Design review of the part built by this model. Coordinates are the model's own, in mm. A direction names the side the tool comes from. Give positions to 0.01 mm unless a question says otherwise; leave off trailing zeros. Loops run counter-clockwise (first coordinate to the right, second up) from the corner with the lowest first, then second, coordinate; pieces in that order, holes last.
from build123d import *

# Parameters (mm, degrees)
ESQUISSE1_W              = 44
ESQUISSE1_H              = 25
BOSS_EXTRU_1_DEPTH       = 1.9
ESQUISSE2_W              = 18
ESQUISSE2_H              = 21.4
ESQUISSE2_W_2            = 12.9
ESQUISSE2_H_2            = 20.7
ENL_V_MAT_EXTRU_1_DEPTH  = 1.1
ESQUISSE3_W              = 9
ESQUISSE3_H              = 12
ENL_V_MAT_EXTRU_2_DEPTH  = 10
ESQUISSE4_W              = 3.5
ESQUISSE4_H              = 6.801352385
ENL_V_MAT_EXTRU_3_DEPTH  = 1.4
ENL_V_MAT_EXTRU_4_DEPTH  = 2.4
ESQUISSE6_W              = 9
ESQUISSE6_H              = 0.8
BOSS_EXTRU_2_DEPTH       = 1
ESQUISSE7_W              = 2
ESQUISSE7_H              = 1.1
BOSS_EXTRU_3_DEPTH       = 1
BOSS_EXTRU_4_DEPTH       = 1
ESQUISSE12_W             = 26.5
ESQUISSE12_H             = 1.9
BOSS_EXTRU_6_DEPTH       = 1
ESQUISSE13_W             = 44
ESQUISSE13_H             = 1
BOSS_EXTRU_7_DEPTH       = 4.9
ESQUISSE14_W             = 44
ESQUISSE14_H             = 27
BOSS_EXTRU_8_DEPTH       = 0.8
ESQUISSE15_W             = 9
ESQUISSE15_H             = 1
ENL_V_MAT_EXTRU_5_DEPTH  = 0.2
ESQUISSE16_W             = 0.8
ESQUISSE16_H             = 1.1
ENL_V_MAT_EXTRU_7_DEPTH  = 2
ESQUISSE18_W             = 1.9
ESQUISSE18_H             = 3.15
ENL_V_MAT_EXTRU_8_DEPTH  = 2
ESQUISSE19_W             = 1
ESQUISSE19_H             = 25
BOSS_EXTRU_10_DEPTH      = 4.9
ENL_V_MAT_EXTRU_9_DEPTH  = 1
ESQUISSE21_W             = 1.9
ESQUISSE21_H             = 2.150656269
BOSS_EXTRU_11_DEPTH      = 17.5
BOSS_EXTRU_12_DEPTH      = 1.1
BOSS_EXTRU_13_DEPTH      = 1.1
ESQUISSE26_W             = 12.9
ESQUISSE26_H             = 17.5
ENL_V_MAT_EXTRU_10_DEPTH = 1.1
ESQUISSE28_W             = 4.9
ESQUISSE28_H             = 25
ENL_V_MAT_EXTRU_12_DEPTH = 10
ESQUISSE30_W             = 4.9
ESQUISSE30_H             = 25
BOSS_EXTRU_14_DEPTH      = 1
ESQUISSE31_W             = 4.9
ESQUISSE31_H             = 4.778042902
ESQUISSE31_H_2           = 4.777647835
ENL_V_MAT_EXTRU_13_DEPTH = 11
ESQUISSE32_W             = 2
ESQUISSE32_H             = 1.1
ENL_V_MAT_EXTRU_14_DEPTH = 5
ESQUISSE33_W             = 4.880014168
ESQUISSE33_H             = 9.610289291
ENL_V_MAT_EXTRU_15_DEPTH = 5
ESQUISSE34_W             = 1.1
ESQUISSE34_H             = 10.612062874
ENL_V_MAT_EXTRU_16_DEPTH = 5
ESQUISSE35_W             = 1.1
ESQUISSE35_H             = 16.502088347
BOSS_EXTRU_15_DEPTH      = 0.1
ESQUISSE36_W             = 1.95
ESQUISSE36_H             = 2.065080621
ESQUISSE36_W_2           = 1.843442291
BOSS_EXTRU_16_DEPTH      = 1
ESQUISSE40_W             = 3.7
ESQUISSE40_H             = 6.2
ENL_V_MAT_EXTRU_18_DEPTH = 1
ESQUISSE39_W             = 7.2
ESQUISSE39_H             = 3
ENL_V_MAT_EXTRU_20_DEPTH = 1
ESQUISSE41_W             = 1.072034993
ESQUISSE41_H             = 2.997764605
ESQUISSE41_W_2           = 1.033542433
BOSS_EXTRU_17_DEPTH      = 0.2
ESQUISSE42_W             = 1.1
ESQUISSE42_H             = 9.602531403
ENL_V_MAT_EXTRU_21_DEPTH = 0.2


with BuildPart() as part:
    # Esquisse1 → Boss.-Extru.1 (new body)
    with BuildSketch(Plane.XY):
        Rectangle(ESQUISSE1_W, ESQUISSE1_H)
    extrude(amount=BOSS_EXTRU_1_DEPTH)

    # Esquisse2 → Enlèv. mat.-Extru.1 (cut)
    with BuildSketch(Plane.XY.offset(1.9)):
        with Locations((-11.5, 1.801352385)):
            Rectangle(ESQUISSE2_W, ESQUISSE2_H)
        with Locations((12.55, -0.999343731)):
            Rectangle(ESQUISSE2_W_2, ESQUISSE2_H_2)
    extrude(amount=-ENL_V_MAT_EXTRU_1_DEPTH, mode=Mode.SUBTRACT)

    # Esquisse3 → Enlèv. mat.-Extru.2 (cut)
    with BuildSketch(Plane.XY.offset(0.8)):
        with Locations((-11.5, 12.5)):
            Rectangle(ESQUISSE3_W, ESQUISSE3_H)
    extrude(amount=-ENL_V_MAT_EXTRU_2_DEPTH, mode=Mode.SUBTRACT)

    # Esquisse4 → Enlèv. mat.-Extru.3 (cut)
    with BuildSketch(Plane.XY.offset(1.9)):
        with Locations((-6.25, -9.099323807)):
            Rectangle(ESQUISSE4_W, ESQUISSE4_H)
    extrude(amount=-ENL_V_MAT_EXTRU_3_DEPTH, mode=Mode.SUBTRACT)

    # Esquisse5 → Enlèv. mat.-Extru.4 (cut)
    with BuildSketch(Plane.XY.offset(1.9)):
        Polygon((-8, -5.698647615), (-14.25, -8.898647615), (-22, -8.898647615), (-22, -12.5), (-4.5, -12.5), (-4.5, -5.698647615), align=None)
    extrude(amount=-ENL_V_MAT_EXTRU_4_DEPTH, mode=Mode.SUBTRACT)

    # Esquisse6 → Boss.-Extru.2 (add)
    with BuildSketch(Plane(origin=(0, 6.5, 0), x_dir=(1, 0, 0), z_dir=(0, 1, 0))):
        with Locations((-11.5, -0.4)):
            Rectangle(ESQUISSE6_W, ESQUISSE6_H)
    extrude(amount=BOSS_EXTRU_2_DEPTH)

    # Esquisse7 → Boss.-Extru.3 (add)
    with BuildSketch(Plane(origin=(0, -8.898647615, 0), x_dir=(1, 0, 0), z_dir=(0, 1, 0))):
        with Locations((-3.5, -1.35)):
            Rectangle(ESQUISSE7_W, ESQUISSE7_H)
    extrude(amount=BOSS_EXTRU_3_DEPTH)

    # Esquisse9 → Boss.-Extru.4 (add)
    with BuildSketch(Plane(origin=(0, 12.5, 0), x_dir=(1, 0, 0), z_dir=(0, 1, 0))):
        Polygon((22, 0), (-2.5, 0), (-7, 0), (-7, -0.8), (-2.5, -0.8), (-2.5, -1.9), (22, -1.9), align=None)
        Polygon((-22, 0), (-20.5, 0), (-16, 0), (-16, -0.8), (-20.5, -0.8), (-20.5, -1.9), (-22, -1.9), align=None)
    extrude(amount=BOSS_EXTRU_4_DEPTH)

    # Esquisse12 → Boss.-Extru.6 (add)
    with BuildSketch(Plane.XZ.offset(12.5)):
        with Locations((8.75, 0.95)):
            Rectangle(ESQUISSE12_W, ESQUISSE12_H)
    extrude(amount=BOSS_EXTRU_6_DEPTH)

    # Esquisse13 → Boss.-Extru.7 (add)
    with BuildSketch(Plane(origin=(0, 0, 0), x_dir=(-1, 0, 0), z_dir=(0, 0, -1))):
        with Locations((0, 13)):
            Rectangle(ESQUISSE13_W, ESQUISSE13_H)
        with Locations((0, -13)):
            Rectangle(ESQUISSE13_W, ESQUISSE13_H)
    extrude(amount=BOSS_EXTRU_7_DEPTH)

    # Esquisse14 → Boss.-Extru.8 (add)
    with BuildSketch(Plane(origin=(0, 0, -4.9), x_dir=(-1, 0, 0), z_dir=(0, 0, -1))):
        Rectangle(ESQUISSE14_W, ESQUISSE14_H)
    extrude(amount=BOSS_EXTRU_8_DEPTH)

    # Esquisse15 → Enlèv. mat.-Extru.5 (cut)
    with BuildSketch(Plane.XY):
        with Locations((-11.5, 13)):
            Rectangle(ESQUISSE15_W, ESQUISSE15_H)
    extrude(amount=-ENL_V_MAT_EXTRU_5_DEPTH, mode=Mode.SUBTRACT)

    # Esquisse16 → Enlèv. mat.-Extru.7 (cut)
    with BuildSketch(Plane.ZY.offset(22)):
        with Locations((-5.3, 11.95)):
            Rectangle(ESQUISSE16_W, ESQUISSE16_H)
    extrude(amount=-ENL_V_MAT_EXTRU_7_DEPTH, mode=Mode.SUBTRACT)

    # Esquisse18 → Enlèv. mat.-Extru.8 (cut)
    with BuildSketch(Plane(origin=(22, 0, 0), x_dir=(0, 0, -1), z_dir=(1, 0, 0))):
        with Locations((-0.95, 10.925)):
            Rectangle(ESQUISSE18_W, ESQUISSE18_H)
    extrude(amount=-ENL_V_MAT_EXTRU_8_DEPTH, mode=Mode.SUBTRACT)

    # Esquisse19 → Boss.-Extru.10 (add)
    with BuildSketch(Plane.XY.offset(-4.9)):
        with Locations((-19.5, 0)):
            Rectangle(ESQUISSE19_W, ESQUISSE19_H)
    extrude(amount=BOSS_EXTRU_10_DEPTH)

    # Esquisse20 → Enlèv. mat.-Extru.9 (cut)
    with BuildSketch(Plane.XY.offset(0.8)):
        Polygon((-4.5, -5.776745759), (-4.5, -3.002088347), (-8.02831202, -3.002088347), (-11.125, -7.298647615), align=None)
    extrude(amount=-ENL_V_MAT_EXTRU_9_DEPTH, mode=Mode.SUBTRACT)

    # Esquisse21 → Boss.-Extru.11 (add)
    with BuildSketch(Plane.ZY.offset(4.5)):
        with Locations((0.95, -12.424671866)):
            Rectangle(ESQUISSE21_W, ESQUISSE21_H)
    extrude(amount=BOSS_EXTRU_11_DEPTH)

    # Esquisse23 → Boss.-Extru.12 (add)
    with BuildSketch(Plane.XY.offset(0.8)):
        Polygon((-4.5, -7.898647615), (-11.348803677, -11.349343731), (-4.5, -11.349343731), align=None)
    extrude(amount=BOSS_EXTRU_12_DEPTH)

    # Esquisse25 → Boss.-Extru.13 (add)
    with BuildSketch(Plane.XY.offset(0.8)):
        Polygon((-16, 13.5), (-20.5, 13.5), (-20.5, -8.898647615), (-14.25, -8.898647615), (-11.125, -7.298647615), (-8.02831202, -3.002088347), (-4.5, -3.002088347), (-4.5, -7.898647615), (-2.5, -7.898647615), (-2.5, 13.5), (-7, 13.5), (-7, 7.5), (-16, 7.5), align=None)
    extrude(amount=BOSS_EXTRU_13_DEPTH)

    # Esquisse26 → Enlèv. mat.-Extru.10 (cut)
    with BuildSketch(Plane.XY.offset(1.9)):
        with Locations((-11.5, 4.75)):
            Rectangle(ESQUISSE26_W, ESQUISSE26_H)
    extrude(amount=-ENL_V_MAT_EXTRU_10_DEPTH, mode=Mode.SUBTRACT)

    # Esquisse28 → Enlèv. mat.-Extru.12 (cut)
    with BuildSketch(Plane.ZY.offset(20)):
        with Locations((-2.45, 0)):
            Rectangle(ESQUISSE28_W, ESQUISSE28_H)
    extrude(amount=-ENL_V_MAT_EXTRU_12_DEPTH, mode=Mode.SUBTRACT)

    # Esquisse30 → Boss.-Extru.14 (add)
    with BuildSketch(Plane.ZY.offset(22)):
        with Locations((-2.45, 0)):
            Rectangle(ESQUISSE30_W, ESQUISSE30_H)
    extrude(amount=-BOSS_EXTRU_14_DEPTH)

    # Esquisse31 → Enlèv. mat.-Extru.13 (cut)
    with BuildSketch(Plane(origin=(-21, 0, 0), x_dir=(0, 0, -1), z_dir=(1, 0, 0))):
        with Locations((2.45, 10.110978549)):
            Rectangle(ESQUISSE31_W, ESQUISSE31_H)
        with Locations((2.45, -10.111176083)):
            Rectangle(ESQUISSE31_W, ESQUISSE31_H_2)
    extrude(amount=-ENL_V_MAT_EXTRU_13_DEPTH, mode=Mode.SUBTRACT)

    # Esquisse32 → Enlèv. mat.-Extru.14 (cut)
    with BuildSketch(Plane(origin=(0, 0, -5.7), x_dir=(-1, 0, 0), z_dir=(0, 0, -1))):
        with Locations((21, 9.515350227)):
            Rectangle(ESQUISSE32_W, ESQUISSE32_H)
        with Locations((21, 6.785575873)):
            Rectangle(ESQUISSE32_W, ESQUISSE32_H)
    extrude(amount=-ENL_V_MAT_EXTRU_14_DEPTH, mode=Mode.SUBTRACT)

    # Esquisse33 → Enlèv. mat.-Extru.15 (cut)
    with BuildSketch(Plane.ZY.offset(22)):
        with Locations((-2.440007084, 7.694855354)):
            Rectangle(ESQUISSE33_W, ESQUISSE33_H)
    extrude(amount=-ENL_V_MAT_EXTRU_15_DEPTH, mode=Mode.SUBTRACT)

    # Esquisse34 → Enlèv. mat.-Extru.16 (cut)
    with BuildSketch(Plane.ZY.offset(22)):
        with Locations((-2.596187743, -2.416320728)):
            Rectangle(ESQUISSE34_W, ESQUISSE34_H)
    extrude(amount=-ENL_V_MAT_EXTRU_16_DEPTH, mode=Mode.SUBTRACT)

    # Esquisse35 → Boss.-Extru.15 (add)
    with BuildSketch(Plane.ZY.offset(5.05)):
        with Locations((1.35, 5.248955826)):
            Rectangle(ESQUISSE35_W, ESQUISSE35_H)
    extrude(amount=BOSS_EXTRU_15_DEPTH)

    # Esquisse36 → Boss.-Extru.16 (add)
    with BuildSketch(Plane.XY.offset(0.8)):
        with Locations((-16.975, 7.632540311)):
            Rectangle(ESQUISSE36_W, ESQUISSE36_H)
        with Locations((-6.078278855, 7.632540311)):
            Rectangle(ESQUISSE36_W_2, ESQUISSE36_H)
    extrude(amount=BOSS_EXTRU_16_DEPTH)

    # Esquisse40 → Enlèv. mat.-Extru.18 (cut)
    with BuildSketch(Plane.XY.offset(1.9)):
        with Locations((1.85, 0)):
            Rectangle(ESQUISSE40_W, ESQUISSE40_H)
    extrude(amount=-ENL_V_MAT_EXTRU_18_DEPTH, mode=Mode.SUBTRACT)

    # Esquisse39 → Enlèv. mat.-Extru.20 (cut)
    with BuildSketch(Plane.XY.offset(1.9)):
        with Locations((2.705958025, 12)):
            Rectangle(ESQUISSE39_W, ESQUISSE39_H)
    extrude(amount=-ENL_V_MAT_EXTRU_20_DEPTH, mode=Mode.SUBTRACT)

    # Esquisse41 → Boss.-Extru.17 (add)
    with BuildSketch(Plane.XY.offset(1.9)):
        with Locations((-1.430059472, 12.001117697)):
            Rectangle(ESQUISSE41_W, ESQUISSE41_H)
        with Locations((6.822729242, 12.001117697)):
            Rectangle(ESQUISSE41_W_2, ESQUISSE41_H)
    extrude(amount=BOSS_EXTRU_17_DEPTH)

    # Esquisse42 → Enlèv. mat.-Extru.21 (cut)
    with BuildSketch(Plane.ZY.offset(5.15)):
        with Locations((1.35, 1.799177355)):
            Rectangle(ESQUISSE42_W, ESQUISSE42_H)
    extrude(amount=-ENL_V_MAT_EXTRU_21_DEPTH, mode=Mode.SUBTRACT)


solid = part.part
Q1. Take a section at A-A (z = -4). Give the boundary of the cut face in (x, y), plus the area to 3 significant figures.
Results:
outline: (-22, -13.5) - (22, -13.5) - (22, -12.5) - (-22, -12.5) - close; (-22, -7.72) - (-21, -7.72) - (-21, 2.89) - (-22, 2.89) - close; (-22, 12.5) - (22, 12.5) - (22, 13.5) - (-22, 13.5) - close
area: 98.6 mm2
Q2. Take a section at B-B (y = -2). Give the boundary of the cut face in (x, z).
Results:
outline: (-22, -5.7) - (22, -5.7) - (22, -4.9) - (-21, -4.9) - (-21, -3.15) - (-22, -3.15) - close; (-22, -2.05) - (-21, -2.05) - (-21, 0) - (22, 0) - (22, 1.9) - (19, 1.9) - (19, 0.8) - (6.1, 0.8) - (6.1, 1.9) - (3.7, 1.9) - (3.7, 0.9) - (0, 0.9) - (0, 1.9) - (-4.95, 1.9) - (-4.95, 0.8) - (-17.95, 0.8) - (-17.95, 1.9) - (-22, 1.9) - close
Q3. Take a section at D-D (y = -5.25). Give the boundary of the cut face in (x, z).
Results:
outline: (-22, -5.7) - (22, -5.7) - (22, -4.9) - (-21, -4.9) - (-21, -3.15) - (-22, -3.15) - close; (-22, -2.05) - (-21, -2.05) - (-21, 0) - (-9.65, 0) - (-9.65, 1.9) - (-22, 1.9) - close; (-4.5, 0) - (22, 0) - (22, 1.9) - (19, 1.9) - (19, 0.8) - (6.1, 0.8) - (6.1, 1.9) - (-4.5, 1.9) - close
Q4. Tool access review of faces 4 (the face through (-6.2, -3.002, 0.5)), 5 (the face through (-21.5, -7.722, -1)), 6 (the face through (-21, 11.4, -5.3)): name each direction out of +Z, -Z, +X, -X, +Y, -Y from which nothing blocks a thin tool from reaching the whole face with its end or side.
Results:
face 4: +Z
face 5: +X, -X
face 6: -Z, -X
Q5. Insertion check: pin 1 (10 mm diameter, centred on x = -4.5, y = -6.5, fed in from +Z); pin 2 (1.5 mm diameter, centred on y = -5.5, z = -1.5, fed in from +X); pin 3 (1.1 mm diameter, centred on x = -6.5, z = 1.5, fed in from +Y); pin 4 (1.5 mm diameter, centred on y = 7, z = -1.5, fed in from +X). Each pin has a flat end and moves straight along its axis. Give the tip position at first contact, or say it passes through.
Results:
pin 1: stops at z = 1.9
pin 2: stops at x = -21
pin 3: stops at y = 8.67
pin 4: passes through
Q6. Wall thickness on line 1 (X direction, y = 0, z = 1.25); line 2 (Z direction, x = -15.5, y = 5); line 3 (Y direction, x = -6, z = -2.75): over which ranges is each line inside the solid? List them lowest first.
Results:
line 1: x = -22 to -17.95, -4.95 to 0, 3.7 to 6.1, 19 to 22
line 2: z = -5.7 to -4.9, 0 to 0.8
line 3: y = -13.5 to -12.5, 12.5 to 13.5
Q7. Take a section at C-C (x = -3). Give the boundary of the cut face in (y, z), plus the area to 3 significant figures.
Results:
outline: (-13.5, -5.7) - (13.5, -5.7) - (13.5, 1.9) - (-13.5, 1.9) - close; hole (-12.5, -4.9) - (12.5, -4.9) - (12.5, 0) - (-12.5, 0) - close
area: 82.7 mm2
Q8. Draft analysis for pull direction Y (two halves, no side actions). For faces 1 (the face through (-7, 10, 0.6)), 2 (the face through (0, 13.5, -2)), 3 (the face through (-21, 6.236, -5.3)), state which applies: pulls with the +Y half, pulls with the -Y half, needs draft (parallel to the pull), parting line crosses it, or undercut.
Results:
face 1: needs draft
face 2: pulls with the +Y half
face 3: undercut
